Source: three-view drawing plus pictorial views. Frame: mm from the lowest corner of the part. Give positions to 0.01 mm unless a question says otherwise; leave off trailing zeros. Write each loop counter-clockwise with the first axis right and the second up, starting at its lowest first coordinate (ties: lowest second). Pieces come first, ordered by that corner, then holes.
Q1. Line query: L1, parallel to Y at x = 1.75, z = 2.5; L2, parallel to Z at x = 0.25, y = 1.9; L3, parallel to Y at x = 0.2, z = 3.25 (1 decimal). Output: solid intervals per line, ascending.
Q2. Draft query along Y for the marked faces 1, 2 and 3. Return one class per face: pulls with the +Y half, pulls with the -Y half, needs draft (parallel to the pull), parting line crosses it, or undercut.
Q3. Cut plane C-C on x = 0.8. Return the cut outline in (y, z).
Q4. Cut plane A-A on z = 2.5. Return the cut outline in (x, y).
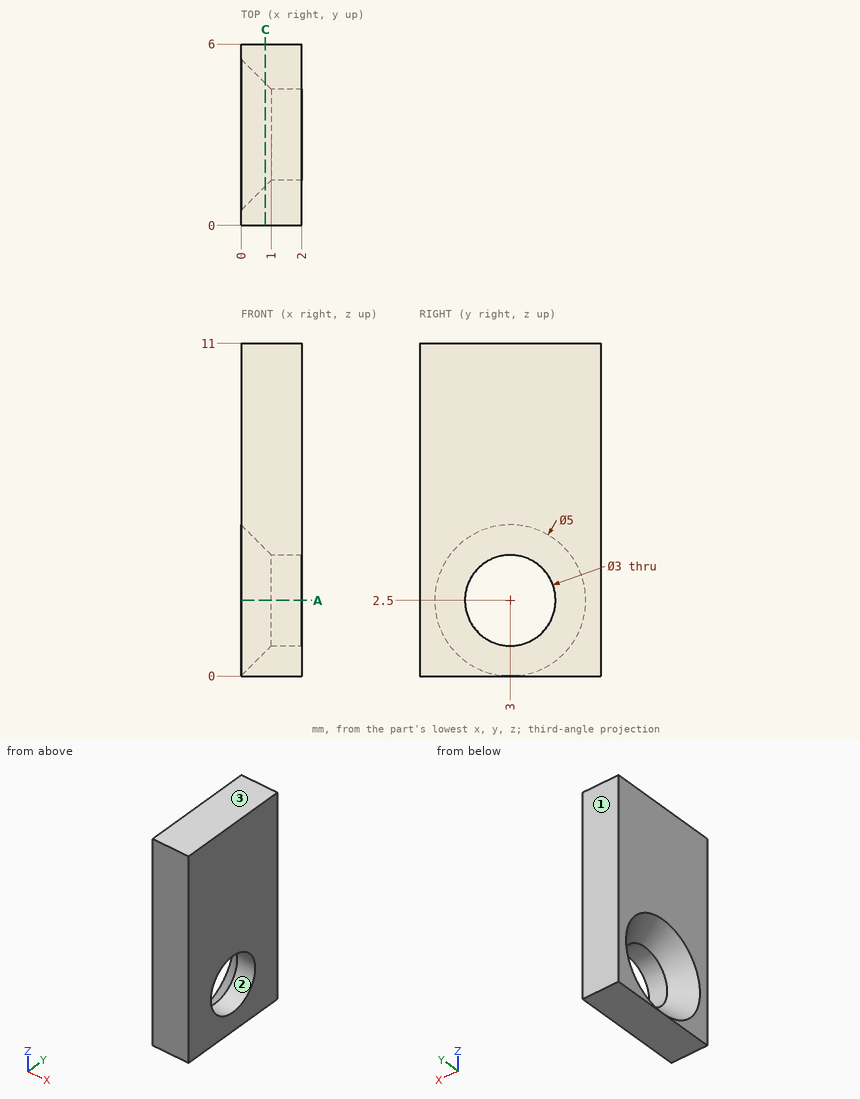
Data:
1. L1: y = 0 to 1.5, 4.5 to 6
1. L2: z = 0 to 0.54, 4.46 to 11
1. L3: y = 0 to 0.8, 5.2 to 6
2. face 1: pulls with the +Y half
2. face 2: undercut
2. face 3: needs draft
3. outline: (0, 0) - (6, 0) - (6, 11) - (0, 11) - close; hole circle Ø3.4 at (3, 2.5)
4. outline: (0, 0) - (2, 0) - (2, 1.5) - (1, 1.5) - (0, 0.5) - close; (0, 5.5) - (1, 4.5) - (2, 4.5) - (2, 6) - (0, 6) - close
